Autodesk Inventor part; units mm, degrees
ref_plane "YZ Plane" through (0, 0, 0) normal (1, 0, 0) x (0, 1, 0)
ref_plane "XZ Plane" through (0, 0, 0) normal (0, 1, 0) x (-1, 0, 0)
ref_plane "XY Plane" through (0, 0, 0) normal (0, 0, 1) x (1, 0, 0)
sketch "Sketch1" plane through (0, 0, 0) normal (0, 0, 1) x (1, 0, 0)
  line L0 (-7.3025, 7.3025) -> (7.3025, 7.3025)
  line L1 (7.3025, 7.3025) -> (7.3025, -7.3025)
  line L2 (7.3025, -7.3025) -> (-7.3025, -7.3025)
  line L3 (-7.3025, -7.3025) -> (-7.3025, 7.3025)
  point P0 (0, 0)
  point P1 (0, 7.3025)
  point P2 (-7.3025, 0)
  dimension "d0" = 14.605
  dimension "d1" = 14.605
extrude "Extrusion1" add sketch "Sketch1" along normal mid plane 25.4
sketch "Sketch2" plane through (-7.3025, -7.3025, 12.7) normal (-1, 0, 0) x (0, 0, 1)
  line L0 (0, 0) -> (0, 14.605)
  line L1 (-25.4, 14.605) -> (0, 14.605)
  line L2 (-25.4, 14.605) -> (-25.4, 0)
  line L3 (0, 0) -> (-25.4, 0)
  line L4 (-19.812, 14.605) -> (-5.588, 14.605)
  line L5 (-5.588, 14.605) -> (-5.588, 0)
  line L6 (-5.588, 0) -> (-19.812, 0)
  line L7 (-19.812, 0) -> (-19.812, 14.605)
  point P0 (-12.7, 0)
  dimension "d4" = 14.224
extrude "Extrusion2" add sketch "Sketch2" along normal blind 6.35 contours L3 L7 L1 L5
sketch "Sketch3" plane through (0, 0, -12.7) normal (0, 0, -1) x (-1, 0, 0)
  line L0 (7.3025, 7.3025) -> (7.3025, -7.3025)
  line L1 (-7.3025, 7.3025) -> (7.3025, 7.3025)
  line L2 (-7.3025, -7.3025) -> (-7.3025, 7.3025)
  line L3 (7.3025, -7.3025) -> (-7.3025, -7.3025)
  circle A0 centre (0, 0) radius 4.3815
  dimension "d7" = 8.763
extrude "Extrusion3" cut sketch "Sketch3" against normal through all contours A0
sketch "Sketch4" plane through (-13.6525, -7.3025, 12.7) normal (-1, 0, 0) x (0, 0, 1)
  circle A0 centre (-12.7, 7.3025) radius 4.3815
  line L0 (-19.812, 0) -> (-19.812, 14.605)
  line L1 (0, 0) -> (-25.4, 0)
  line L2 (-19.812, 14.605) -> (-5.588, 14.605)
  line L3 (-19.812, 0) -> (-19.812, 14.605)
  line L4 (-5.588, 0) -> (-19.812, 0)
  line L5 (-5.588, 14.605) -> (-5.588, 0)
  point P0 (-12.7, 14.605)
  point P1 (-19.812, 7.3025)
  dimension "d10" = 8.763
extrude "Extrusion4" cut sketch "Sketch4" against normal blind 13.7414 contours A0
thread "Thread1"
thread "Thread2"
thread "Thread3"
equation "\"d0\" = d1"
properties part number "2203P-2"
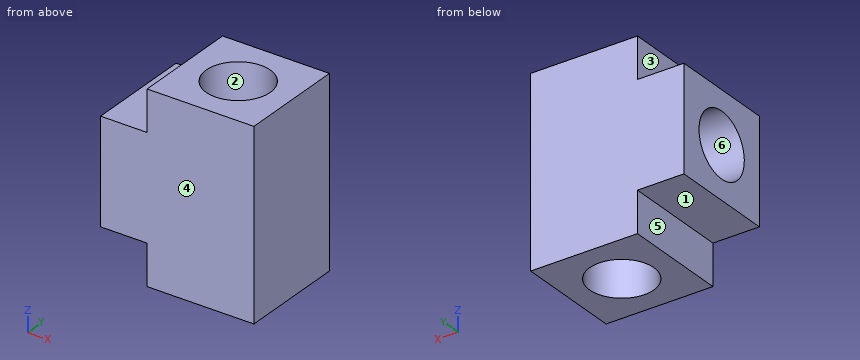
Geometry check sheet. Reference: the model listing, model coordinates, mm. Face numbers are marked on the shaded views. A direction names the side the tool comes from. Give positions to 0.01 mm unless a question says otherwise; leave off trailing zeros. Loops run counter-clockwise (first coordinate to the right, second up) from the corner with the lowest first, then second, coordinate; pieces in that order, holes last. Notation, with made-up numbers: (22, -35) -> (51, -35) arc R20 cw to (51, -27) -> close; hole circle Ø2 at (69, -21.5). An arc over 180 degrees is marked (long way). Answer in a Markdown table with one row per item. Add a question column.
1) Cross-section at A-A on y = 0. Record the boundary of the cut face in (x, z).
2) Set-up check for the marked faces 1, 2 and 3: record each of +Z, -Z, +X, -X, +Y, -Y from which the full face is reachable in a straight line by a thin tool's end or side.
3) Cross-section at B-B on z = -8. Record the boundary of the cut face in (x, y), and give its area (3 significant figures).
4) Material ranges on probe 1 along Y at (x, z) = (-5.5, 0); probe 2 along X at (y, z) = (0.25, 7.5); probe 3 along X at (y, z) = (2.5, -6.5), recorded low to high. Write a range as from..to.
5) Cross-section at D-D on x = -6. Record the boundary of the cut face in (y, z).
6) Gauge pin test, flat ends, axial feed: P1, Ø4.5, axis at y = 0, z = 9.5, coming from the -X side; P2, Ø7, axis at x = -11.5, y = 0, coming from the -Z side; P3, Ø5.5, axis at x = 0, y = 0, coming from the +Z side; P4, Ø7, axis at x = -11, y = 1, coming from the +Z side. Record the tip position at first contact, or that the pin passes through.
7) Draft check along Y on the marked faces 4, 5 and 6. Enter one of: pulls with the +Y half, pulls with the -Y half, needs draft (parallel to the pull), parting line crosses it, or undercut.
8) Cross-section at C-C on x = -2.5. Record the boundary of the cut face in (y, z).
Outcome:
| question | item | result |
|---|---|---|
| 1 | outline | (-13.65, -7.11) -> (-7.3, -7.11) -> (-7.3, -12.7) -> (-4.38, -12.7) -> (-4.38, -4.38) -> (-13.65, -4.38) -> close; (-13.65, 4.38) -> (-4.38, 4.38) -> (-4.38, 12.7) -> (-7.3, 12.7) -> (-7.3, 7.11) -> (-13.65, 7.11) -> close; (4.38, -12.7) -> (7.3, -12.7) -> (7.3, 12.7) -> (4.38, 12.7) -> close |
| 2 | face 1 | -Z, -X, +Y, -Y |
| 2 | face 2 | +Z, -Z |
| 2 | face 3 | +Z, -X, +Y, -Y |
| 3 | outline | (-7.3, -7.3) -> (7.3, -7.3) -> (7.3, 7.3) -> (-7.3, 7.3) -> close; hole circle Ø8.76 at (0, 0) |
| 3 | area | 153 mm^2 |
| 4 | probe 1 | y = -7.3..-4.38, 4.38..7.3 |
| 4 | probe 2 | x = -7.3..-4.37, 4.37..7.3 |
| 4 | probe 3 | x = -13.65..-3.6, 3.6..7.3 |
| 5 | outline | (-7.3, -12.7) -> (7.3, -12.7) -> (7.3, 12.7) -> (-7.3, 12.7) -> close; hole circle Ø8.76 at (0, 0) |
| 6 | P1 | stops at x = -7.3 |
| 6 | P2 | stops at z = -7.11 |
| 6 | P3 | passes through |
| 6 | P4 | stops at z = 7.11 |
| 7 | face 4 | pulls with the -Y half |
| 7 | face 5 | needs draft |
| 7 | face 6 | undercut |
| 8 | outline | (-7.3, -12.7) -> (-3.6, -12.7) -> (-3.6, -2.5) arc R4.38 cw to (-3.6, 2.5) -> (-3.6, 12.7) -> (-7.3, 12.7) -> close; (3.6, -12.7) -> (7.3, -12.7) -> (7.3, 12.7) -> (3.6, 12.7) -> (3.6, 2.5) arc R4.38 cw to (3.6, -2.5) -> close |
